For this review, use the dimensioned drawing (mm, ordinates from the lowest corner) and the shaded views. Round coordinates to 2 decimals unless told otherwise and drop trailing zeros. Order: outer loops, then holes, each group sorted by start corner. A loop starts at its lowest first (then second) coordinate and runs counter-clockwise, first axis right, second up. Notation, with made-up numbers: (67.5, 60.5) -> (96.5, 60.5) arc R17 ccw to (96.5, 67.5) -> close; hole circle Ø5 at (3, 49). An arc over 180 degrees is marked (long way). Answer in a Markdown table with one row per item.
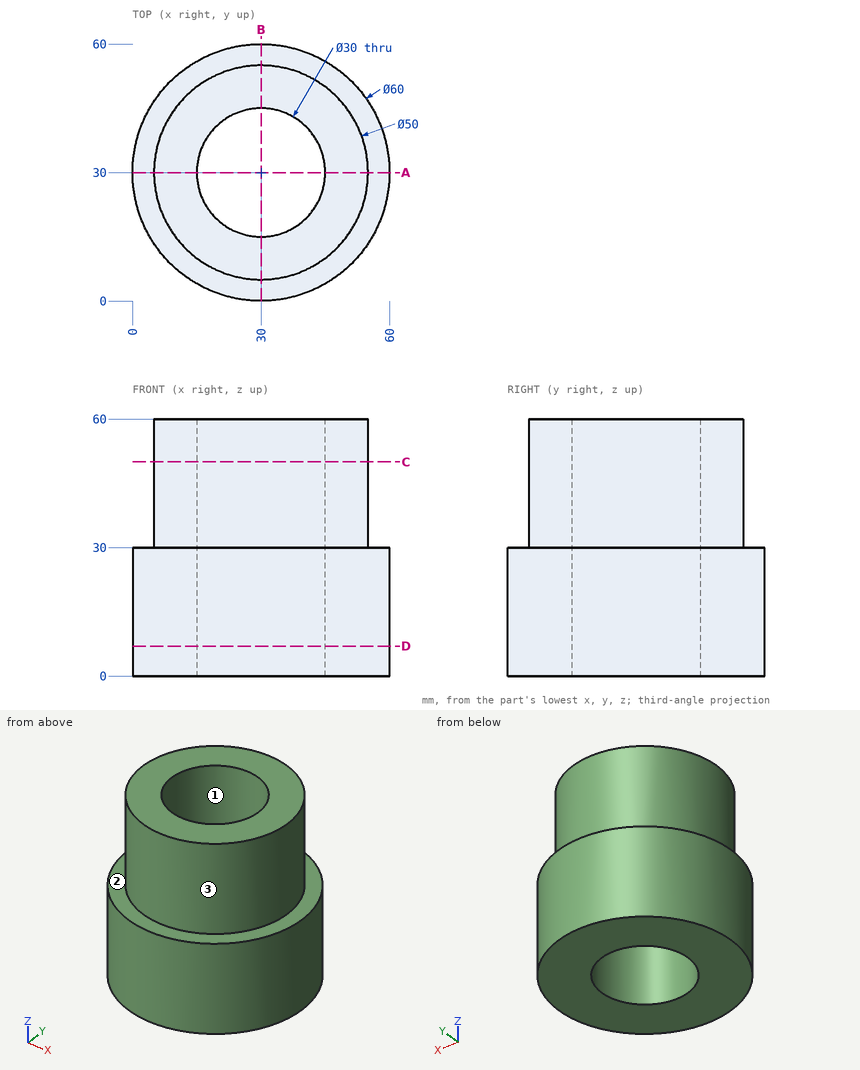
Q1. Take a section at C-C, the plane z = 50. Write out the cut boundary in (x, y), then the cut area to 3 significant figures.
Answer key:
| item | result |
|---|---|
| outline | circle Ø50 at (30, 30); hole circle Ø30 at (30, 30) |
| area | 1,260 mm^2 |
Q2. Clearance check with flat-ended pins moving along their axes: pin 1 Ø1 at (y, z) = (49.5, 35) entering from -X; pin 2 Ø6 at (x, z) = (52.5, 36.5) entering from +Y; pin 3 Ø5 at (x, z) = (41.5, 38) entering from -Y. State where each tip first meets the part, or that it passes through.
Answer key:
| item | result |
|---|---|
| pin 1 | stops at x = 13.75 |
| pin 2 | stops at y = 45.64 |
| pin 3 | stops at y = 6.68 |
Q3. To check wall thickness, follow probe 1 along Y at (x, z) = (30, 42.5); probe 2 along Y at (x, z) = (30, 26); probe 3 along Z at (x, y) = (56.5, 30). State the ranges of each line that lie inside material, in increasing order.
Answer key:
| item | result |
|---|---|
| probe 1 | y = 5 to 15, 45 to 55 |
| probe 2 | y = 0 to 15, 45 to 60 |
| probe 3 | z = 0 to 30 |
Q4. Take a section at D-D, the plane z = 7. Write out the cut boundary in (x, y).
Answer key:
| item | result |
|---|---|
| outline | circle Ø60 at (30, 30); hole circle Ø30 at (30, 30) |
Q5. Take a section at A-A, the plane y = 30. Write out the cut boundary in (x, z).
Answer key:
| item | result |
|---|---|
| outline | (0, 0) -> (15, 0) -> (15, 60) -> (5, 60) -> (5, 30) -> (0, 30) -> close; (45, 0) -> (60, 0) -> (60, 30) -> (55, 30) -> (55, 60) -> (45, 60) -> close |
Q6. The part is to be moulded in two halves that separate along X. For the marked faces 1, 2 and 3, say which applies: +X half, -X half, draft (parallel to the pull), parting line (faces both ways), or undercut.
Answer key:
| item | result |
|---|---|
| face 1 | undercut |
| face 2 | draft |
| face 3 | parting line |
